Here's the drawing with two shaded views (mm, measured from the low corner). I have some questions. A direction names the side the tool comes from. Give positions to 0.01 mm unless a question says otherwise; leave off trailing zeros. Order: outer loops, then holes, each group sorted by start corner. A loop starts at its lowest first (then second) coordinate and runs counter-clockwise, first axis right, second up. Notation, with made-up numbers: M 72.5,-36 L 111.5,-36 A11 cw 111.5,-32 Z; hole C -24,79 d3. An arc over 180 degrees is marked long. Write each question's results on one line, items separated by ' | '.
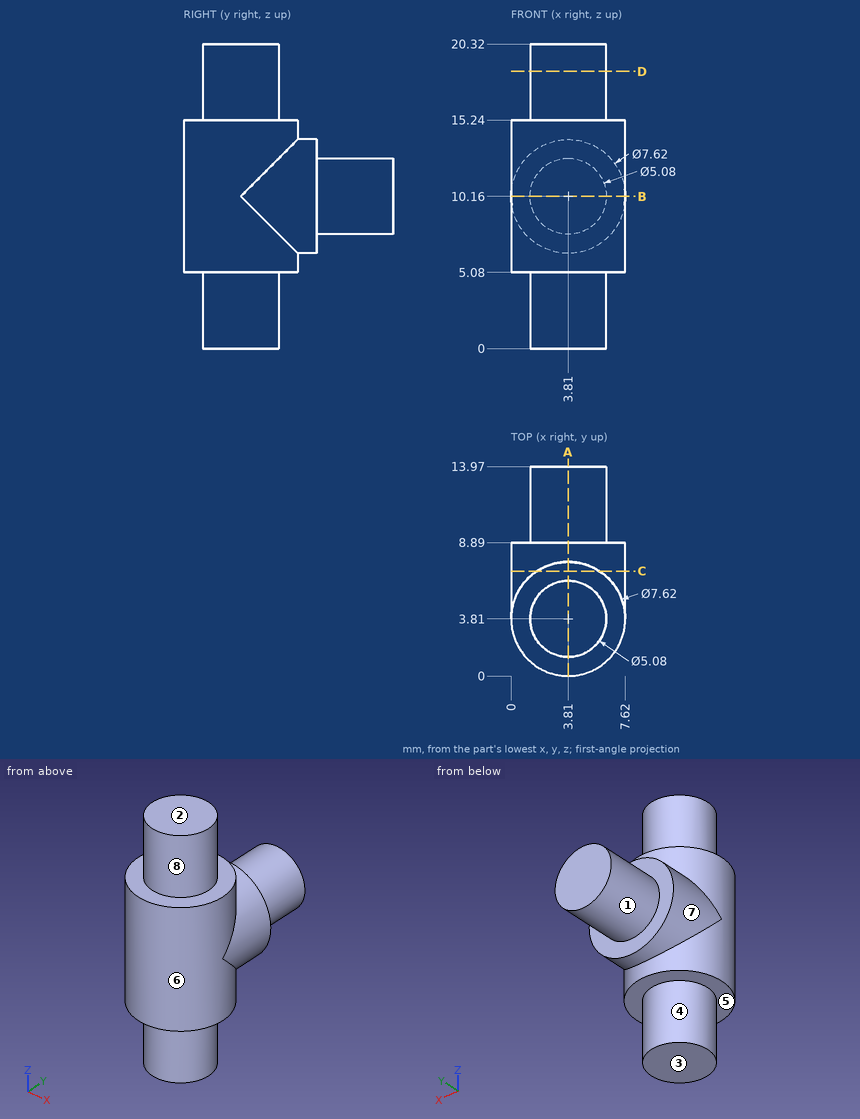
(1) Imagine slicing it at D-D, the plane z = 18.5. Write out the boundary of the cut face in (x, y).
Data:
outline: C 3.81,3.81 d5.08
(2) Imagine slicing it at C-C, the plane y = 7. Write out the boundary of the cut face in (x, z).
Data:
outline: M 1.73,5.08 L 5.89,5.08 L 5.89,6.97 A3.81 ccw 5.89,13.35 L 5.89,15.24 L 1.73,15.24 L 1.73,13.35 A3.81 ccw 1.73,6.97 Z
(3) Will this pin go through, and if not, where does the flat tip stop? P1, Ø3, axis at x = 6, y = 7.5, coming from the -Z side.
Data:
P1: stops at z = 5.08
(4) We'd pull the mould along Z, two halves only. Please class the marked faces 1, 2, 3 and 4: +Z half, -Z half, draft (parallel to the pull), parting line (faces both ways), or undercut.
Data:
face 1: parting line | face 2: +Z half | face 3: -Z half | face 4: draft
(5) I need wall thicknesses on L1, parallel to X at y = 4, z = 5.5; L2, parallel to Y at x = 4, z = 8; L3, parallel to Z at x = 1.5, y = 1.5. Which ranges of each line are inside material? Lowest first, please. Write a range as from..to.
Data:
L1: x = 0..7.62 | L2: y = 0..13.97 | L3: z = 5.08..15.24
(6) For the marked faces 5, 6, 7 and 8, which set-ups out of +Z, -Z, +X, -X, +Y, -Y let a thin tool reach every point of the face, with its end or its side?
Data:
face 5: -Z | face 6: none | face 7: +Y | face 8: +Z
(7) Imagine slicing it at A-A, the plane x = 3.81. Write out the boundary of the cut face in (y, z).
Data:
outline: M 0,5.08 L 1.27,5.08 L 1.27,0 L 6.35,0 L 6.35,5.08 L 7.62,5.08 L 7.62,6.35 L 8.89,6.35 L 8.89,7.62 L 13.97,7.62 L 13.97,12.7 L 8.89,12.7 L 8.89,13.97 L 7.62,13.97 L 7.62,15.24 L 6.35,15.24 L 6.35,20.32 L 1.27,20.32 L 1.27,15.24 L 0,15.24 Z
(8) Imagine slicing it at B-B, the plane z = 10.16. Write out the boundary of the cut face in (x, y), plus the area to 3 significant figures.
Data:
outline: M 0,3.81 A3.81 ccw 7.62,3.81 L 7.62,8.89 L 6.35,8.89 L 6.35,13.97 L 1.27,13.97 L 1.27,8.89 L 0,8.89 Z | area: 87.3 mm2
